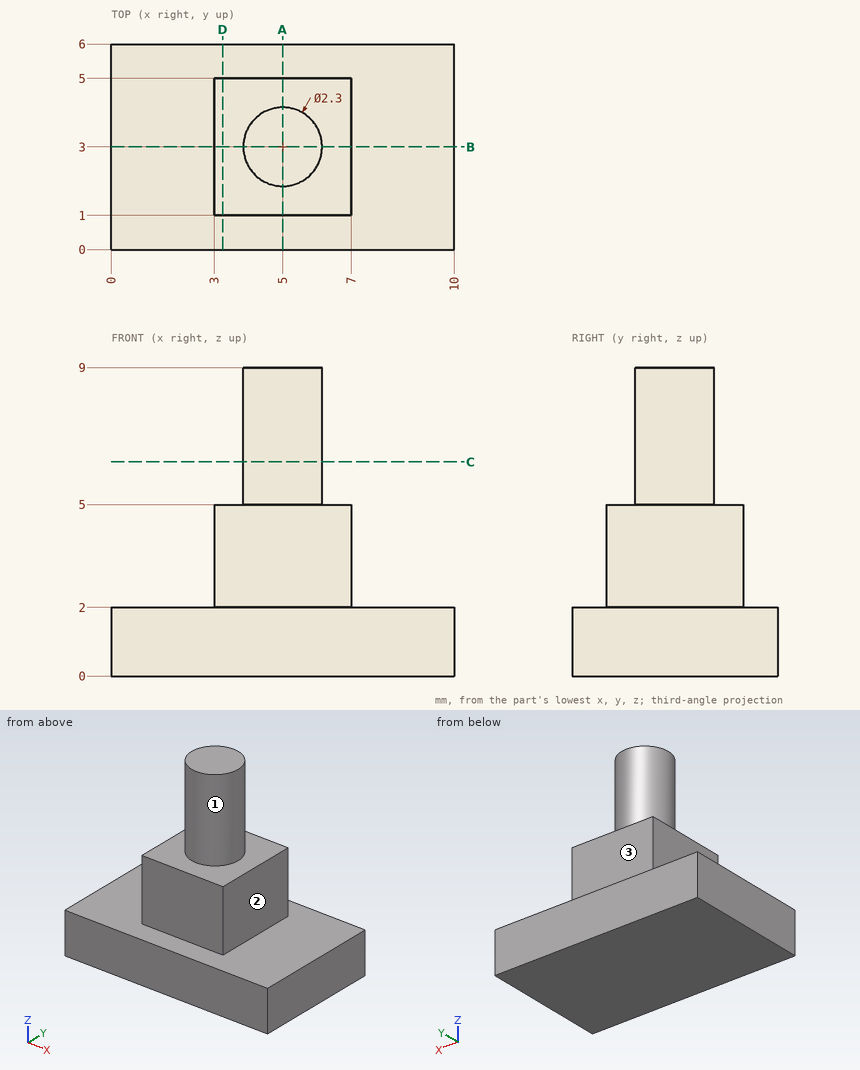
Print and shaded views of the part. All mm, measured from the part's lowest x, y and z. A direction names the side the tool comes from. Coordinates: 2 decimals unless noted, no trailing zeros. Write each loop counter-clockwise with the first axis right and the second up, starting at its lowest first coordinate (ties: lowest second). Pieces come first, ordered by that corner, then holes. Notation, with made-up numbers: (46, 0) -> (54, 0) arc R29 ccw to (54, 35) -> close; hole circle Ø6 at (-27, 55.25). An arc over 180 degrees is marked (long way). Use CSV: the item, a comma, the result in double quotes. Start each with the question number.
Q1. Drill centre lines: probe 1 along Z at (x, y) = (1.5, 3.35); probe 2 along Z at (x, y) = (6, 4.35); probe 3 along X at (y, z) = (1.6, 3). Where is each one in solid material? Low to high.
Q2. Cut at B-B, the plane y = 3. List the corners of the cut face in (x, z), then the cut area to 3 significant figures.
Q3. Cut at D-D, the plane x = 3.25. List the corners of the cut face in (y, z), then the cut area to 3 significant figures.
Q4. Cut at A-A, the plane x = 5. List the corners of the cut face in (y, z), then the cut area to 3 significant figures.
Q5. Cut at C-C, the plane z = 6.25. List the corners of the cut face in (x, y), then the cut area to 3 significant figures.
Q6. 3-axis set-ups, long thin cutter, end or side, ignore diameter. For the marked faces 1, 2 and 3: which of +Z, -Z, +X, -X, +Y, -Y reach the whole face in a straight line?
Q7. Flat gauge pins, fed straight in: pin 1 Ø2.5 at (x, z) = (4.5, 4) entering from -Y; pin 2 Ø0.9 at (y, z) = (3.5, 3) entering from +X. Where does each tip first touch, or does it go through?
Checked values:
1,probe 1,"z = 0 to 2"
1,probe 2,"z = 0 to 5"
1,probe 3,"x = 3 to 7"
2,outline,"(0, 0) -> (10, 0) -> (10, 2) -> (7, 2) -> (7, 5) -> (6.15, 5) -> (6.15, 9) -> (3.85, 9) -> (3.85, 5) -> (3, 5) -> (3, 2) -> (0, 2) -> close"
2,area,"41.2 mm²"
3,outline,"(0, 0) -> (6, 0) -> (6, 2) -> (5, 2) -> (5, 5) -> (1, 5) -> (1, 2) -> (0, 2) -> close"
3,area,"24.0 mm²"
4,outline,"(0, 0) -> (6, 0) -> (6, 2) -> (5, 2) -> (5, 5) -> (4.15, 5) -> (4.15, 9) -> (1.85, 9) -> (1.85, 5) -> (1, 5) -> (1, 2) -> (0, 2) -> close"
4,area,"33.2 mm²"
5,outline,"circle Ø2.3 at (5, 3)"
5,area,"4.15 mm²"
6,face 1,"+Z"
6,face 2,"+Z, +X, +Y, -Y"
6,face 3,"+Z, +X, -X, +Y"
7,pin 1,"stops at y = 1"
7,pin 2,"stops at x = 7"
